CAD build for the part. Positions are in the model's coordinates, mm. A direction names the side the tool comes from. Give positions to 0.01 mm unless a question says otherwise; leave off trailing zeros. Loops run counter-clockwise (first coordinate to the right, second up) from the corner with the lowest first, then second, coordinate; pieces in that order, holes last. Notation, with made-up numbers: M 21.5,21 L 35.5,21 A26 ccw 35.5,49 Z; hole C 49,-28.5 d10. An arc over 180 degrees is marked long. One line per question, with ' | ' between items.
```python
from build123d import *

# Parameters (mm, degrees)
BOSS_EXTRUDE1_DEPTH              = 12.7
HOLE3_D                          = 3.175
HOLE3_DEPTH                      = 31.75
HOLE3_CSINK_D                    = 10.16
HOLE3_CSINK_ANGLE                = 82
HOLE3_TIP                        = 0.953866233
HOLE6_D                          = 3.175
HOLE6_DEPTH                      = 38.1
HOLE6_CSINK_D                    = 10.16
HOLE6_CSINK_ANGLE                = 82
HOLE6_TIP                        = 0.953866233
HOLE7_D                          = 3.175
HOLE7_DEPTH                      = 31.75
HOLE7_CSINK_D                    = 10.16
HOLE7_CSINK_ANGLE                = 82
HOLE7_TIP                        = 0.953866233
HOLE8_D                          = 3.175
HOLE8_DEPTH                      = 31.75
HOLE8_CSINK_D                    = 10.16
HOLE8_CSINK_ANGLE                = 82
HOLE8_TIP                        = 0.953866233
F_15_64_0_23438_DIAMETER_HOLE1_D = 5.953252
F_15_64_0_23438_DIAMETER_HOLE2_D = 5.953252
CUT_EXTRUDE1_DEPTH               = 334.311975083
FILLET1_R                        = 38.1


with BuildPart() as part:
    # Sketch1 → Boss-Extrude1 (new body)
    with BuildSketch(Plane.XY):
        Polygon((-88.190159952, 0), (-222.052967181, 0), (-222.052967181, -248.25), (-64.977416983, -197.966048293), align=None)
    extrude(amount=-BOSS_EXTRUDE1_DEPTH)

    # Hole3
    with Locations(Plane(origin=(-234.752967181, 1073.364195846, -135.816741379), x_dir=(0, 0, -1), z_dir=(-1, 0, 0))):
        with Locations((-129.466741379, 1300.662770337), (-129.466741379, 1128.612770337), (129.198788767, 1128.612770337), (129.198788767, 1300.662770337)):
            CounterSinkHole(HOLE3_D / 2, HOLE3_CSINK_D / 2, depth=HOLE3_DEPTH, counter_sink_angle=HOLE3_CSINK_ANGLE)
            with Locations((0, 0, -(HOLE3_DEPTH + HOLE3_TIP / 2))):  # 118° drill point
                Cone(0, HOLE3_D / 2, HOLE3_TIP, mode=Mode.SUBTRACT)

    # Hole6
    with Locations(Plane(origin=(181.039434513, 1073.364195846, 0), x_dir=(-0.9271838545667885, -0.3746065934159093, 0), z_dir=(0, 0, 1))):
        with Locations((707.166557203, 1065.270372796), (674.127983646, 944.603090451)):
            CounterSinkHole(HOLE6_D / 2, HOLE6_CSINK_D / 2, depth=HOLE6_DEPTH, counter_sink_angle=HOLE6_CSINK_ANGLE)
            with Locations((0, 0, -(HOLE6_DEPTH + HOLE6_TIP / 2))):  # 118° drill point
                Cone(0, HOLE6_D / 2, HOLE6_TIP, mode=Mode.SUBTRACT)

    # Hole7
    with Locations(Plane(origin=(181.039434513, 12.7, -135.816741379), x_dir=(0, 0, -1), z_dir=(0, 1, 0))):
        with Locations((129.198788767, 384.042401694), (-129.466741379, 384.042401694), (-129.466741379, 304.786761906), (-110.416741379, 409.442401694), (-0.133976306, 409.442401694), (110.148788767, 409.442401694), (129.198788767, 304.786761906)):
            CounterSinkHole(HOLE7_D / 2, HOLE7_CSINK_D / 2, depth=HOLE7_DEPTH, counter_sink_angle=HOLE7_CSINK_ANGLE)
            with Locations((0, 0, -(HOLE7_DEPTH + HOLE7_TIP / 2))):  # 118° drill point
                Cone(0, HOLE7_D / 2, HOLE7_TIP, mode=Mode.SUBTRACT)

    # Hole8
    with Locations(Plane(origin=(531.197640696, -20.449854654, -135.816741379), x_dir=(0, 0, 1), z_dir=(0.3048844921716131, -0.9523893355310409, 0))):
        with Locations((-129.257383629, 761.035393152), (129.466741379, 663.01461615), (129.466741379, 760.835922116), (-129.408220012, 663.214203478)):
            CounterSinkHole(HOLE8_D / 2, HOLE8_CSINK_D / 2, depth=HOLE8_DEPTH, counter_sink_angle=HOLE8_CSINK_ANGLE)
            with Locations((0, 0, -(HOLE8_DEPTH + HOLE8_TIP / 2))):  # 118° drill point
                Cone(0, HOLE8_D / 2, HOLE8_TIP, mode=Mode.SUBTRACT)

    # 15/64 (0.23438) Diameter Hole1 (through all)
    with Locations(Plane.XY):
        with Locations((-117.397327374, -12.17947903), (-209.352967162, -12.179479032)):
            Hole(F_15_64_0_23438_DIAMETER_HOLE1_D / 2)

    # 15/64 (0.23438) Diameter Hole2 (through all)
    with Locations(Plane.XY):
        with Locations((-209.352967181, -170.846075828)):
            Hole(F_15_64_0_23438_DIAMETER_HOLE2_D / 2)

    # Sketch22 → Cut-Extrude1 (cut, through all)
    with BuildSketch(Plane.XY):
        Polygon((-99.555964999, -175.698330504), (-116.434796625, -31.75), (-190.302967181, -31.75), (-190.302967181, -204.748796153), align=None)
    extrude(amount=-CUT_EXTRUDE1_DEPTH, mode=Mode.SUBTRACT)

    # Fillet1
    fillet1_edges = [part.edges().sort_by_distance(p)[0] for p in [
        (-99.555964999, -175.698330504, -6.35),
        (-190.302967181, -204.748796153, -6.35),
        (-190.302967181, -31.75, -6.35),
        (-116.434796625, -31.75, -6.35),
    ]]
    fillet(fillet1_edges, radius=FILLET1_R)


solid = part.part
```
Item 1: Drill centre lines: line 1 along X through (y, z) = (-170.5, -11); line 2 along X through (y, z) = (-97, -4.5); line 3 along X through (y, z) = (-64, -2). Where is each one in solid material? Low to high. Write a range as [from, to].
Conclusion:
line 1: [-222.05, -212.31], [-206.4, -185.81], [-109.61, -68.2] | line 2: [-222.05, -190.3], [-108.78, -76.82] | line 3: [-222.05, -189.85], [-112.68, -80.69]
Item 2: Saw through at D-D on y = -218.5. Give the cut face in (x, z), and give its area (3 significant figures).
Conclusion:
outline: M -222.05,-12.7 L -129.12,-12.7 L -129.12,0 L -222.05,0 Z | area: 1,180 mm²
Item 3: Mould opens along X. For faces 3 (the flat face through (-222.053, -122, -6)), 4 (the flat face through (-154, 0, -6)), 5 (the cylindrical face through (-178.846, -42.615, -6.439)), 6 (the cylindrical face through (-208.965, -167.895, -6.439)) say: pulls with the +X half, pulls with the -X half, needs draft (parallel to the pull), parting line crosses it, or undercut.
Conclusion:
face 3: pulls with the -X half | face 4: needs draft | face 5: undercut | face 6: undercut
Item 4: 3-axis set-ups, long thin cutter, end or side, ignore diameter. For faces 1 (the flat face through (-144.61, -223.46, -6.26)), 2 (the cylindrical face through (-108.82, -169.295, -6.439)): which of +Z, -Z, +X, -X, +Y, -Y reach the whole face in a straight line?
Conclusion:
face 1: +Z, -Z, +X, -Y | face 2: +Z, -Z
Item 5: Saw through at C-C on z = -10. State how many separate pieces and enclosed holes the cut face has, and give its area (3 significant figures).
Conclusion:
separate pieces: 1 | enclosed holes: 6 | area: 20,800 mm²
Item 6: Saw through at B-B on y = -95.5. Give the cut face in (x, z).
Conclusion:
outline: M -222.05,-12.7 L -190.3,-12.7 L -190.3,0 L -222.05,0 Z; M -108.96,-12.7 L -76.99,-12.7 L -76.99,0 L -108.96,0 Z
Item 7: Drop flat-ended pins along their axis: P1, Ø2.5, axis at x = -123.75, z = -6.35, coming from the +Y side; P2, Ø5, axis at x = -90.15, y = -54.99, coming from the +Z side; P3, Ø1, axis at x = -145, z = -9, coming from the -Y side. Give the stop position or say it passes through.
Conclusion:
P1: y = -19.25 | P2: z = -2.96 | P3: y = -223.74
Item 8: Saw through at A-A on x = -170. Give the cut face in (y, z).
Conclusion:
outline: M -231.59,-12.7 L -186.24,-12.7 L -186.24,0 L -231.59,0 Z; M -36.16,-12.7 L 0,-12.7 L 0,0 L -36.16,0 Z
